from build123d import *

# Parameters (mm, degrees)
F0_R     = 1.5
F1_DEPTH = 3


with BuildPart() as f1:
    # F0 (on Right) → F1 (new body)
    with BuildSketch(Plane.YZ):
        Polygon((113.5, 122), (113.5, 125), (83.5, 125), (83.5, 122), (48.5, 122), (48.5, 125), (18.5, 125), (18.5, 122), (-16.5, 122), (-16.5, 125), (-46.5, 125), (-46.5, 122), (-86.5, 122), (-153.5, -55), (-153.5, -125), (153.5, -125), (153.5, 122), align=None)
        with Locations((-137.5, -109)):
            Circle(F0_R, mode=Mode.SUBTRACT)
        with Locations((-138.5, -71)):
            Circle(F0_R, mode=Mode.SUBTRACT)
        with Locations((137.5, -109)):
            Circle(F0_R, mode=Mode.SUBTRACT)
        with Locations((-66.5, 110)):
            Circle(F0_R, mode=Mode.SUBTRACT)
        with Locations((137.5, 109)):
            Circle(F0_R, mode=Mode.SUBTRACT)
    extrude(amount=F1_DEPTH)


solid = f1.part
Design review of the part built by this model. Coordinates are the model's own, in mm. Give positions to 0.01 mm unless a question says otherwise; leave off trailing zeros. Write each loop counter-clockwise with the first axis right and the second up, starting at its lowest first coordinate (ties: lowest second). Pieces come first, ordered by that corner, then holes. Notation, with made-up numbers: M 18,-21 L 52,-21 A24 ccw 52,3 Z; hole C 26.5,62 d4. An arc over 180 degrees is marked long. Answer as a JSON object with one key per item and string values. Group by question number.
1) Mouldability with a two-part tool opening along X and no side actions: class faces 1 (the face through (3, -2, 2)), 2 (the face through (1.48, -119.53, 34.74)), 3 (the face through (0, -2, 2)) as released by +X, released by -X, zero draft, split by the parting line, or undercut.
2) We need section C-C (y = -105.5). Give the boundary of the cut face in (x, z), and give its area (3 significant figures).
3) Clearance check with flat-ended pins moving along their axes: pin 1 Ø0.9 at (x, y) = (2, -6.5) entering from +Z; pin 2 Ø1.5 at (x, z) = (2, 123.5) entering from -Y; pin 3 Ø0.9 at (x, z) = (1.5, 123.5) entering from +Y. State where each tip first meets the part, or that it passes through.
4) We need section B-B (z = 83.5). Give the boundary of the cut face in (x, y).
5) For line 1 along Y through (x, z) = (2.05, -109); line 2 along Z through (x, y) = (1.1, 137.5); line 3 along Z through (x, y) = (1.2, -66.5), list the stretches that pass through material, from the lowest coordinate up.
6) We need section A-A (x = 2.1). Give the boundary of the cut face in (y, z), and give its area (3 significant figures).
Answer key:
{
 "1": {"face 1": "released by +X", "face 2": "zero draft", "face 3": "released by -X"},
 "2": {"outline": "M 0,-125 L 3,-125 L 3,71.81 L 0,71.81 Z", "area": "590 mm²"},
 "3": {"pin 1": "stops at z = 122", "pin 2": "stops at y = -46.5", "pin 3": "stops at y = 113.5"},
 "4": {"outline": "M 0,-101.07 L 3,-101.07 L 3,153.5 L 0,153.5 Z"},
 "5": {"line 1": "y = -153.5 to -139, -136 to 136, 139 to 153.5", "line 2": "z = -125 to -110.5, -107.5 to 107.5, 110.5 to 122", "line 3": "z = -125 to 108.5, 111.5 to 122"},
 "6": {"outline": "M -153.5,-125 L 153.5,-125 L 153.5,122 L 113.5,122 L 113.5,125 L 83.5,125 L 83.5,122 L 48.5,122 L 48.5,125 L 18.5,125 L 18.5,122 L -16.5,122 L -16.5,125 L -46.5,125 L -46.5,122 L -86.5,122 L -153.5,-55 Z; hole C -138.5,-71 d3; hole C -137.5,-109 d3; hole C -66.5,110 d3; hole C 137.5,-109 d3; hole C 137.5,109 d3", "area": "70,100 mm²"}
}
